```python
from build123d import *

# Parameters (mm, degrees)
SKETCH1_W                       = 320
SKETCH1_H                       = 220
THE_UPPER_CHASISS_DEPTH         = 1.25
BATTARY_REACH                   = 196.169
SKETCH2_R                       = 3.5
BATTARY_DIRECTION_2_REACH       = 196.169
POWER_SECTION_REACH             = 196.169
SKETCH3_R                       = 3.5
POWER_SECTION_DIRECTION_2_REACH = 196.169
ARDUINO_R                       = 3.5
ARDUINO_SECTION_DEPTH           = 2.5
SKETCH7_R                       = 5
LINK_NAILS_DEPTH                = 2.5
SKETCH9_W                       = 20
SKETCH9_H                       = 40
RECT_CUT_DEPTH                  = 2.5
SKETCH10_R                      = 12.759028862
CIRC_CUT_DEPTH                  = 2.5
FILLET4_START                   = -2
FILLET4_DEPTH                   = 4


with BuildPart() as part:
    # Sketch1 → the upper chasiss (new, symmetric)
    with BuildSketch(Plane(origin=(0, 0, 0), x_dir=(1, 0, 0), z_dir=(0, 1, 0))):
        Rectangle(SKETCH1_W, SKETCH1_H)
    extrude(amount=THE_UPPER_CHASISS_DEPTH, both=True)

    # Battary: up to this face of the body (flat: up to its plane)
    battary_end = Plane(part.part.faces().sort_by_distance((0, 1.25, 0))[0])
    # Sketch2 → Battary (cut, up to the picked face)
    with BuildSketch(Plane(origin=(0, 0, 0), x_dir=(1, 0, 0), z_dir=(0, 1, 0)), mode=Mode.PRIVATE) as battary_sk1:
        with Locations(Location((70, 0, 0), (0, 0, 90))):
            Circle(SKETCH2_R)
    battary_tool1 = split(extrude(battary_sk1.sketch, amount=BATTARY_REACH, mode=Mode.PRIVATE), bisect_by=battary_end, keep=Keep.BOTH, mode=Mode.PRIVATE)
    # Sketch2 → Battary (cut, up to the picked face)
    with BuildSketch(Plane(origin=(0, 0, 0), x_dir=(1, 0, 0), z_dir=(0, 1, 0)), mode=Mode.PRIVATE) as battary_sk2:
        with Locations(Location((45, 0, 0), (0, 0, 90))):
            Circle(SKETCH2_R)
    battary_tool2 = split(extrude(battary_sk2.sketch, amount=BATTARY_REACH, mode=Mode.PRIVATE), bisect_by=battary_end, keep=Keep.BOTH, mode=Mode.PRIVATE)
    add(battary_tool1.solids().sort_by(Axis((70, 0, 0), (0, 1, 0)))[0], mode=Mode.SUBTRACT)
    add(battary_tool2.solids().sort_by(Axis((45, 0, 0), (0, 1, 0)))[0], mode=Mode.SUBTRACT)

    # Battary direction 2: up to this face of the body (flat: up to its plane)
    battary_direction_2_end = Plane(part.part.faces().sort_by_distance((0, -1.25, 0))[0])
    # Sketch2 → Battary direction 2 (cut, up to the picked face)
    with BuildSketch(Plane(origin=(0, 0, 0), x_dir=(1, 0, 0), z_dir=(0, 1, 0)), mode=Mode.PRIVATE) as battary_direction_2_sk1:
        with Locations(Location((70, 0, 0), (0, 0, 90))):
            Circle(SKETCH2_R)
    battary_direction_2_tool1 = split(extrude(battary_direction_2_sk1.sketch, amount=-BATTARY_DIRECTION_2_REACH, mode=Mode.PRIVATE), bisect_by=battary_direction_2_end, keep=Keep.BOTH, mode=Mode.PRIVATE)
    # Sketch2 → Battary direction 2 (cut, up to the picked face)
    with BuildSketch(Plane(origin=(0, 0, 0), x_dir=(1, 0, 0), z_dir=(0, 1, 0)), mode=Mode.PRIVATE) as battary_direction_2_sk2:
        with Locations(Location((45, 0, 0), (0, 0, 90))):
            Circle(SKETCH2_R)
    battary_direction_2_tool2 = split(extrude(battary_direction_2_sk2.sketch, amount=-BATTARY_DIRECTION_2_REACH, mode=Mode.PRIVATE), bisect_by=battary_direction_2_end, keep=Keep.BOTH, mode=Mode.PRIVATE)
    add(battary_direction_2_tool1.solids().sort_by(Axis((70, 0, 0), (0, -1, 0)))[0], mode=Mode.SUBTRACT)
    add(battary_direction_2_tool2.solids().sort_by(Axis((45, 0, 0), (0, -1, 0)))[0], mode=Mode.SUBTRACT)

    # power section: up to this face of the body (flat: up to its plane)
    power_section_end = Plane(part.part.faces().sort_by_distance((-0.062934128, -1.25, 0))[0])
    # Sketch3 → power section (cut, up to the picked face)
    with BuildSketch(Plane(origin=(0, 0, 0), x_dir=(1, 0, 0), z_dir=(0, 1, 0)), mode=Mode.PRIVATE) as power_section_sk1:
        with Locations(Location((-56.898371951, -47.760148577, 0), (0, 0, 90))):
            Circle(SKETCH3_R)
    power_section_tool1 = split(extrude(power_section_sk1.sketch, amount=-POWER_SECTION_REACH, mode=Mode.PRIVATE), bisect_by=power_section_end, keep=Keep.BOTH, mode=Mode.PRIVATE)
    # Sketch3 → power section (cut, up to the picked face)
    with BuildSketch(Plane(origin=(0, 0, 0), x_dir=(1, 0, 0), z_dir=(0, 1, 0)), mode=Mode.PRIVATE) as power_section_sk2:
        with Locations(Location((-16.898371951, -47.760148577, 0), (0, 0, 90))):
            Circle(SKETCH3_R)
    power_section_tool2 = split(extrude(power_section_sk2.sketch, amount=-POWER_SECTION_REACH, mode=Mode.PRIVATE), bisect_by=power_section_end, keep=Keep.BOTH, mode=Mode.PRIVATE)
    # Sketch3 → power section (cut, up to the picked face)
    with BuildSketch(Plane(origin=(0, 0, 0), x_dir=(1, 0, 0), z_dir=(0, 1, 0)), mode=Mode.PRIVATE) as power_section_sk3:
        with Locations(Location((-56.898371951, -87.760148577, 0), (0, 0, 90))):
            Circle(SKETCH3_R)
    power_section_tool3 = split(extrude(power_section_sk3.sketch, amount=-POWER_SECTION_REACH, mode=Mode.PRIVATE), bisect_by=power_section_end, keep=Keep.BOTH, mode=Mode.PRIVATE)
    add(power_section_tool1.solids().sort_by(Axis((-56.898372, 0, 47.760149), (0, -1, 0)))[0], mode=Mode.SUBTRACT)
    add(power_section_tool2.solids().sort_by(Axis((-16.898372, 0, 47.760149), (0, -1, 0)))[0], mode=Mode.SUBTRACT)
    add(power_section_tool3.solids().sort_by(Axis((-56.898372, 0, 87.760149), (0, -1, 0)))[0], mode=Mode.SUBTRACT)

    # power section direction 2: up to this face of the body (flat: up to its plane)
    power_section_direction_2_end = Plane(part.part.faces().sort_by_distance((-0.062934128, 1.25, 0))[0])
    # Sketch3 → power section direction 2 (cut, up to the picked face)
    with BuildSketch(Plane(origin=(0, 0, 0), x_dir=(1, 0, 0), z_dir=(0, 1, 0)), mode=Mode.PRIVATE) as power_section_direction_2_sk1:
        with Locations(Location((-56.898371951, -47.760148577, 0), (0, 0, 90))):
            Circle(SKETCH3_R)
    power_section_direction_2_tool1 = split(extrude(power_section_direction_2_sk1.sketch, amount=POWER_SECTION_DIRECTION_2_REACH, mode=Mode.PRIVATE), bisect_by=power_section_direction_2_end, keep=Keep.BOTH, mode=Mode.PRIVATE)
    # Sketch3 → power section direction 2 (cut, up to the picked face)
    with BuildSketch(Plane(origin=(0, 0, 0), x_dir=(1, 0, 0), z_dir=(0, 1, 0)), mode=Mode.PRIVATE) as power_section_direction_2_sk2:
        with Locations(Location((-16.898371951, -47.760148577, 0), (0, 0, 90))):
            Circle(SKETCH3_R)
    power_section_direction_2_tool2 = split(extrude(power_section_direction_2_sk2.sketch, amount=POWER_SECTION_DIRECTION_2_REACH, mode=Mode.PRIVATE), bisect_by=power_section_direction_2_end, keep=Keep.BOTH, mode=Mode.PRIVATE)
    # Sketch3 → power section direction 2 (cut, up to the picked face)
    with BuildSketch(Plane(origin=(0, 0, 0), x_dir=(1, 0, 0), z_dir=(0, 1, 0)), mode=Mode.PRIVATE) as power_section_direction_2_sk3:
        with Locations(Location((-56.898371951, -87.760148577, 0), (0, 0, 90))):
            Circle(SKETCH3_R)
    power_section_direction_2_tool3 = split(extrude(power_section_direction_2_sk3.sketch, amount=POWER_SECTION_DIRECTION_2_REACH, mode=Mode.PRIVATE), bisect_by=power_section_direction_2_end, keep=Keep.BOTH, mode=Mode.PRIVATE)
    add(power_section_direction_2_tool1.solids().sort_by(Axis((-56.898372, 0, 47.760149), (0, 1, 0)))[0], mode=Mode.SUBTRACT)
    add(power_section_direction_2_tool2.solids().sort_by(Axis((-16.898372, 0, 47.760149), (0, 1, 0)))[0], mode=Mode.SUBTRACT)
    add(power_section_direction_2_tool3.solids().sort_by(Axis((-56.898372, 0, 87.760149), (0, 1, 0)))[0], mode=Mode.SUBTRACT)

    # arduino → arduino section (cut, symmetric)
    with BuildSketch(Plane(origin=(0, 0, 0), x_dir=(1, 0, 0), z_dir=(0, 1, 0))):
        with Locations(Location((-77.933527642, 82.588848983, 0), (0, 0, 90))):
            Circle(ARDUINO_R)
        with Locations(Location((-77.933527642, 32.588848983, 0), (0, 0, 90))):
            Circle(ARDUINO_R)
        with Locations(Location((-27.933527642, 67.388848983, 0), (0, 0, 90))):
            Circle(ARDUINO_R)
        with Locations(Location((-27.933527642, 40.388848983, 0), (0, 0, 90))):
            Circle(ARDUINO_R)
    extrude(amount=ARDUINO_SECTION_DEPTH, both=True, mode=Mode.SUBTRACT)

    # Sketch7 → link nails (cut, symmetric)
    with BuildSketch(Plane(origin=(0, 1.25, 0), x_dir=(1, 0, 0), z_dir=(0, 1, 0))):
        with Locations(Location((-122.762547967, -90.864975812, 0), (0, 0, 270))):
            Circle(SKETCH7_R)
        with Locations(Location((-122.762547967, 90.864975812, 0), (0, 0, 90))):
            Circle(SKETCH7_R)
        with Locations(Location((122.762547967, -90.864975812, 0), (0, 0, 90))):
            Circle(SKETCH7_R)
        with Locations(Location((122.762547967, 90.864975812, 0), (0, 0, 270))):
            Circle(SKETCH7_R)
    extrude(amount=LINK_NAILS_DEPTH, both=True, mode=Mode.SUBTRACT)

    # Sketch9 → rect cut (cut, symmetric)
    with BuildSketch(Plane(origin=(0, 1.25, 0), x_dir=(1, 0, 0), z_dir=(0, 1, 0))):
        with Locations((126.210934146, 0)):
            Rectangle(SKETCH9_W, SKETCH9_H)
    extrude(amount=RECT_CUT_DEPTH, both=True, mode=Mode.SUBTRACT)

    # Sketch10 → circ cut (cut, symmetric)
    with BuildSketch(Plane(origin=(0, 1.25, 0), x_dir=(1, 0, 0), z_dir=(0, 1, 0))):
        with Locations(Location((-35.518377642, -13.276286789, 0), (0, 0, 270))):
            Circle(SKETCH10_R)
    extrude(amount=CIRC_CUT_DEPTH, both=True, mode=Mode.SUBTRACT)

    # Fillet4: read off the stored shape, not the designer's step
    # Fillet4 outline → Fillet4 (cut)
    with BuildSketch(Plane(origin=(0, 0, 0), x_dir=(1, 0, 0), z_dir=(0, 1, 0)).offset(FILLET4_START)):
        with BuildLine():
            Line((-160, -110), (-110, -110))
            add(Edge.make_bspline(
                [(-110, -110), (-160, -110), (-160, -60)],
                knots=[0, 0, 0, 1, 1, 1], degree=2, weights=[1, 0.707106781, 1]))
            Line((-160, -60), (-160, -110))
        make_face()
        with BuildLine():
            add(Edge.make_bspline(
                [(160, -60), (160, -110), (110, -110)],
                knots=[0, 0, 0, 1, 1, 1], degree=2, weights=[1, 0.707106781, 1]))
            Line((110, -110), (160, -110))
            Line((160, -110), (160, -60))
        make_face()
        with BuildLine():
            Line((-160, 110), (-160, 60))
            add(Edge.make_bspline(
                [(-160, 60), (-160, 110), (-110, 110)],
                knots=[0, 0, 0, 1, 1, 1], degree=2, weights=[1, 0.707106781, 1]))
            Line((-110, 110), (-160, 110))
        make_face()
        with BuildLine():
            add(Edge.make_bspline(
                [(110, 110), (160, 110), (160, 60)],
                knots=[0, 0, 0, 1, 1, 1], degree=2, weights=[1, 0.707106781, 1]))
            Line((160, 60), (160, 110))
            Line((160, 110), (110, 110))
        make_face()
    extrude(amount=FILLET4_DEPTH, mode=Mode.SUBTRACT)


solid = part.part
```
Here's how the part is built. I have some questions about the finished solid (model axes, mm). Give positions to 0.01 mm unless a question says otherwise; leave off trailing zeros. Loops run counter-clockwise (first coordinate to the right, second up) from the corner with the lowest first, then second, coordinate; pieces in that order, holes last. Notation, with made-up numbers: M -27,-28.75 L 1,-28.75 A31 cw 1,2.25 Z; hole C 78,50 d9. An arc over 180 degrees is marked long. Use one line per item in the form item = value. Start each with the question number.
Q1. If we section it at A-A (x = 45): Write out the boundary of the cut face in (y, z).
Q2. Thinking about a two-plate mould opening in X: for faces 1 (the flat face through (-2, 1.25, -2)), 2 (the cylindrical face through (41.53, 0.02, 0.46)), which applies, +X half, -X half, draft (parallel to the pull), parting line (faces both ways), or undercut?
Q3. Will these pins go through, and if not, where does the flat tip stop? pin 1 Ø11 at (x, z) = (70, 0) entering from -Y; pin 2 Ø6.5 at (x, z) = (45, 0) entering from +Y; pin 3 Ø1.2 at (x, y) = (129.5, 0) entering from -Z; pin 4 Ø1.2 at (x, y) = (126, 0.5) entering from +Z.
Q4. I need wall thicknesses on line 1 along X through (y, z) = (-1, -17); line 2 along Z through (x, y) = (45, -0.55); line 3 along Z through (x, y) = (-20, -0.6). Which ranges of each line are inside material? Lowest first, please.
Q5. If we section it at C-C (y = 0.6): State how many separate pieces and enclosed holes the cut face has, then the cut area to 3 significant figures.
Q6. If we section it at B-B (z = 10.5): Write out the boundary of the cut face in (x, y).
Taken from the geometry:
q1.outline = M -1.25,-110 L 1.25,-110 L 1.25,-3.5 L -1.25,-3.5 Z; M -1.25,3.5 L 1.25,3.5 L 1.25,110 L -1.25,110 Z
q2.face_1 = draft
q2.face_2 = undercut
q3.pin_1 = -1.25
q3.pin_2 = through
q3.pin_3 = -106.29
q3.pin_4 = 107.57
q4.line_1 = -160 to 116.21, 136.21 to 160
q4.line_2 = -110 to -3.5, 3.5 to 110
q4.line_3 = -110 to 46.14, 49.38 to 110
q5.separate_pieces = 1
q5.enclosed_holes = 15
q5.area = 66,300 mm^2
q6.outline = M -160,-1.25 L -47.97,-1.25 L -47.97,1.25 L -160,1.25 Z; M -23.07,-1.25 L 116.21,-1.25 L 116.21,1.25 L -23.07,1.25 Z; M 136.21,-1.25 L 160,-1.25 L 160,1.25 L 136.21,1.25 Z
